Build history of the part. All positions in model axes, mm. A direction names the side the tool comes from. Give positions to 0.01 mm unless a question says otherwise; leave off trailing zeros. Loops run counter-clockwise (first coordinate to the right, second up) from the corner with the lowest first, then second, coordinate; pieces in that order, holes last.
1) Flat gauge pins, fed straight in: P1, Ø1, axis at y = 8.42, z = 6.94, coming from the +X side; P2, Ø0.5, axis at x = 1, z = 7, coming from the -Y side; P3, Ø3, axis at y = 9, z = 5, coming from the +X side; P4, Ø2, axis at x = 10.41, z = 7.11, coming from the +Y side. Where does each tip first touch, or does it go through?
2) Band-saw the part on B-B on z = 7.25. List the corners of the cut face in (x, y).
3) Band-saw the part on D-D on z = 4.75. List the corners of the cut face in (x, y), then the cut area to 3 significant figures.
4) Band-saw the part on A-A on x = 10. List the corners of the cut face in (y, z), then the cut area to 3 significant figures.
5) Wall check: line 1 (Z direction, x = 4, y = 8); line 2 (X direction, y = 23.5, z = 4.5); line 3 (Y direction, x = 7.5, z = 10.5). Give the ranges that are in metal, low to high.
6) 3-axis set-ups, long thin cutter, end or side, ignore diameter. For faces 1 (the flat face through (1, 1.483, 7)), 2 (the flat face through (1.843, 14, 7)), 3 (the flat face through (7, 14.06, 13.29)): which of +Z, -Z, +X, -X, +Y, -Y reach the whole face in a straight line?
7) Band-saw the part on C-C on y = 13. List the corners of the cut face in (x, z), then the cut area to 3 significant figures.
8) Two-plate mould, pull along Z, no slides. Class faces 4 (the cylindrical face through (0.909, 18.727, 6.833)), 5 (the flat face through (5, 10, 0)), 6 (the flat face through (7, 14.06, 0.91)): +Z half, -Z half, draft (parallel to the pull), parting line (faces both ways), or undercut.
```python
from build123d import *

# Parameters (mm, degrees)
BOSS_EXTRUDE1_DEPTH = 14.224
SKETCH2_W           = 10.456669683
SKETCH2_H           = 10.544
CUT_EXTRUDE1_DEPTH  = 24.807321
SKETCH3_R           = 0.8509
CUT_EXTRUDE2_DEPTH  = 10
SKETCH4_R           = 0.8509
CUT_EXTRUDE3_DEPTH  = 1.482678733


with BuildPart() as part:
    # Sketch1 → Boss-Extrude1 (new body)
    with BuildSketch(Plane.XY):
        Polygon((1.843330317, 26.29), (12.3, 1.482678733), (12.3, 0), (0, 0), (0, 26.29), align=None)
    extrude(amount=BOSS_EXTRUDE1_DEPTH)

    # Sketch2 → Cut-Extrude1 (cut)
    with BuildSketch(Plane(origin=(0, 26.29, 0), x_dir=(1, 0, 0), z_dir=(0, 1, 0))):
        with Locations((7.071665159, -7.112)):
            Rectangle(SKETCH2_W, SKETCH2_H)
    extrude(amount=-CUT_EXTRUDE1_DEPTH, mode=Mode.SUBTRACT)

    # Sketch3 → Cut-Extrude2 (cut)
    with BuildSketch(Plane.ZY):
        with Locations((6.943990858, 17.883471262)):
            Circle(SKETCH3_R)
        with Locations((6.943990858, 8.417089843)):
            Circle(SKETCH3_R)
    extrude(amount=-CUT_EXTRUDE2_DEPTH, mode=Mode.SUBTRACT)

    # Sketch4 → Cut-Extrude3 (cut)
    with BuildSketch(Plane.XZ):
        with Locations(Location((10.409934908, 7.112, 0), (0, 0, 270))):
            Circle(SKETCH4_R)
        with Locations(Location((0.943553489, 7.112, 0), (0, 0, 270))):
            Circle(SKETCH4_R)
    extrude(amount=-CUT_EXTRUDE3_DEPTH, mode=Mode.SUBTRACT)


solid = part.part
```
Findings below:
1. P1: passes through
1. P2: stops at y = 1.48
1. P3: stops at x = 1.84
1. P4: stops at y = 1.48
2. outline: (0, 0) - (0.1, 0) - (0.1, 1.48) - (1.78, 1.48) - (1.78, 0) - (9.57, 0) - (9.57, 1.48) - (1.84, 1.48) - (1.84, 7.62) - (0, 7.62) - close; (0, 9.21) - (1.84, 9.21) - (1.84, 17.09) - (0, 17.09) - close; (0, 18.68) - (1.84, 18.68) - (1.84, 26.29) - (0, 26.29) - close; (11.25, 0) - (12.3, 0) - (12.3, 1.48) - (11.25, 1.48) - close
3. outline: (0, 0) - (12.3, 0) - (12.3, 1.48) - (1.84, 1.48) - (1.84, 26.29) - (0, 26.29) - close
3. area: 64.0 mm2
4. outline: (0, 0) - (6.94, 0) - (6.94, 1.84) - (1.48, 1.84) - (1.48, 6.37) - (0, 6.37) - close; (0, 7.86) - (1.48, 7.86) - (1.48, 12.38) - (6.94, 12.38) - (6.94, 14.22) - (0, 14.22) - close
4. area: 39.0 mm2
5. line 1: z = 0 to 1.84, 12.38 to 14.22
5. line 2: x = 0 to 1.84
5. line 3: y = 0 to 1.48
6. face 1: -Y
6. face 2: +X, +Y
6. face 3: +Z, -Z, +X, +Y
7. outline: (0, 0) - (7.45, 0) - (7.45, 1.84) - (1.84, 1.84) - (1.84, 12.38) - (7.45, 12.38) - (7.45, 14.22) - (0, 14.22) - close
7. area: 46.8 mm2
8. face 4: undercut
8. face 5: -Z half
8. face 6: draft
